Geometry check sheet. Reference: the model listing, model coordinates, mm. Face numbers are marked on the shaded views. A direction names the side the tool comes from. Give positions to 0.01 mm unless a question says otherwise; leave off trailing zeros. Order: outer loops, then holes, each group sorted by start corner. A loop starts at its lowest first (then second) coordinate and runs counter-clockwise, first axis right, second up. Notation, with made-up numbers: (-33, 67) - (-6, 67) arc R27 ccw to (-6, 98) - close; hole circle Ø5 at (-3.75, 8.5). An arc over 180 degrees is marked (long way). Put each result on its own line as item: value. Start each with the question number.
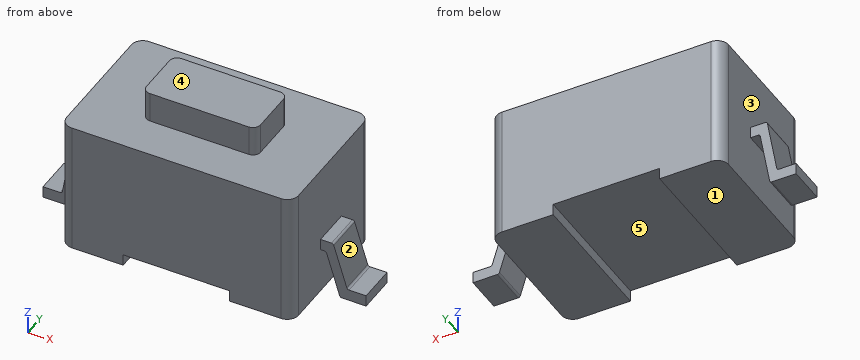
```python
from build123d import *

# Parameters (mm, degrees)
SKETCH001_W  = 6.1
SKETCH001_H  = 3.7
PAD001_DEPTH = 3.5
SKETCH002_W  = 2.8
SKETCH002_H  = 3.7
POCKET_DEPTH = 0.3
FILLET_R     = 0.3
SKETCH003_W  = 3
SKETCH003_H  = 1.5
PAD002_DEPTH = 0.8
FILLET001_R  = 0.2
PAD_DEPTH    = 0.5


with BuildPart() as obj1:
    # Sketch001 → Pad001 (new body)
    with BuildSketch(Plane.XY):
        Rectangle(SKETCH001_W, SKETCH001_H)
    extrude(amount=PAD001_DEPTH)

    # Sketch002 → Pocket (cut)
    with BuildSketch(Plane(origin=(0, 0, 0), x_dir=(1, 0, 0), z_dir=(0, 0, -1))):
        Rectangle(SKETCH002_W, SKETCH002_H)
    extrude(amount=-POCKET_DEPTH, mode=Mode.SUBTRACT)

    # Fillet
    fillet_edges = [obj1.edges().sort_by_distance(p)[0] for p in [
        (-3.05, -1.85, 1.75),
        (-3.05, 1.85, 1.75),
        (3.05, -1.85, 1.75),
        (3.05, 1.85, 1.75),
    ]]
    fillet(fillet_edges, radius=FILLET_R)

    # Sketch003 → Pad002 (new body)
    with BuildSketch(Plane.XY.offset(3.5)):
        Rectangle(SKETCH003_W, SKETCH003_H)
    extrude(amount=PAD002_DEPTH)

    # Fillet001
    fillet001_edges = [obj1.edges().sort_by_distance(p)[0] for p in [
        (1.5, -0.75, 3.9),
        (1.5, 0.75, 3.9),
        (-1.5, 0.75, 3.9),
        (-1.5, -0.75, 3.9),
    ]]
    fillet(fillet001_edges, radius=FILLET001_R)


with BuildPart() as fusion:
    # Sketch → Pad (new body, symmetric)
    with BuildSketch(Plane.XZ):
        with BuildLine():
            Line((4.25, 0), (4.25, 0.3))
            Line((4.25, 0.3), (3.8, 0.3))
            ThreePointArc((3.742663, 0.342323), (3.764367, 0.311727), (3.8, 0.3))
            Line((3.742663, 0.342323), (3.398806, 1.457677))
            ThreePointArc((3.398806, 1.457677), (3.377102, 1.488273), (3.341469, 1.5))
            Line((3.341469, 1.5), (3.05, 1.5))
            Line((3.05, 1.5), (3.05, 1.2))
            Line((3.153657, 1.2), (3.05, 1.2))
            ThreePointArc((3.210994, 1.157677), (3.18929, 1.188273), (3.153657, 1.2))
            Line((3.554852, 0.042323), (3.210994, 1.157677))
            ThreePointArc((3.554852, 0.042323), (3.576556, 0.011727), (3.612189, 0))
            Line((4.25, 0), (3.612189, 0))
        make_face()
        with BuildLine():
            Line((-3.05, 1.5), (-3.05, 1.8))
            Line((-3.434818, 1.8), (-3.05, 1.8))
            ThreePointArc((-3.434818, 1.8), (-3.473385, 1.785963), (-3.493906, 1.750419))
            Line((-3.740912, 0.349581), (-3.493906, 1.750419))
            ThreePointArc((-3.8, 0.3), (-3.761433, 0.314037), (-3.740912, 0.349581))
            Line((-4.25, 0.3), (-3.8, 0.3))
            Line((-4.25, 0), (-4.25, 0.3))
            Line((-4.25, 0), (-3.612189, 0))
            ThreePointArc((-3.612189, 0), (-3.573621, 0.014037), (-3.5531, 0.049581))
            Line((-3.5531, 0.049581), (-3.306095, 1.450419))
            ThreePointArc((-3.247006, 1.5), (-3.285573, 1.485963), (-3.306095, 1.450419))
            Line((-3.247006, 1.5), (-3.05, 1.5))
        make_face()
    extrude(amount=PAD_DEPTH, both=True)

    # Fusion: union obj1
    add(obj1.part)


solid = fusion.part
```
Item 1: Release check for a two-part mould opening along X. For the marked faces 1, 2 and 3 record: +X half, -X half, draft (parallel to the pull), parting line (faces both ways), or undercut.
Item 2: Gauge pin test, flat ends, axial feed: pin 1 Ø1.3 at (x, z) = (-3.5, 0.5) entering from +Y; pin 2 Ø0.6 at (x, z) = (-4, 0.5) entering from -Y; pin 3 Ø2 at (x, y) = (0, 0.5) entering from -Z; pin 4 Ø2 at (x, z) = (-3, 0.5) entering from -Y. Record the tip position at first contact, or that the pin passes through.
Item 3: Thickness scan on line 1 along X through (y, z) = (0.35, 0.45); line 2 along X through (y, z) = (1.05, 3.45); line 3 along Z through (x, y) = (-3, 0.4). Record the ranges inside material, lowest first.
Item 4: Cross-section at A-A (z = 3.6). Enter the section's corners in (x, y), and give its area (3 significant figures).
Item 5: Set-up check for the marked faces 4 and 5: record each of +Z, -Z, +X, -X, +Y, -Y from which the full face is reachable in a straight line by a thin tool's end or side.
Item 6: Cross-section at D-D (x = 2). Enter the section's corners in (y, z).
Item 7: Cross-section at B-B (y = -0.95). Enter the section's corners in (x, z), and give its area (3 significant figures).
Item 8: Cross-section at C-C (z = 0.5). Enter the section's corners in (x, y), and give its area (3 significant figures).
Recorded:
1. face 1: draft
1. face 2: +X half
1. face 3: undercut
2. pin 1: stops at y = 1.83
2. pin 2: stops at y = -0.5
2. pin 3: stops at z = 0.3
2. pin 4: stops at y = -1.85
3. line 1: x = -3.72 to -3.48, -3.05 to 3.05, 3.43 to 3.71
3. line 2: x = -3.05 to 3.05
3. line 3: z = 0 to 3.5
4. outline: (-1.5, -0.55) arc R0.2 ccw to (-1.3, -0.75) - (1.3, -0.75) arc R0.2 ccw to (1.5, -0.55) - (1.5, 0.55) arc R0.2 ccw to (1.3, 0.75) - (-1.3, 0.75) arc R0.2 ccw to (-1.5, 0.55) - close
4. area: 4.47 mm^2
5. face 4: +Z, +X, -X, +Y, -Y
5. face 5: -Z, +Y, -Y
6. outline: (-1.85, 0) - (1.85, 0) - (1.85, 3.5) - (-1.85, 3.5) - close
7. outline: (-3.05, 0) - (-1.4, 0) - (-1.4, 0.3) - (1.4, 0.3) - (1.4, 0) - (3.05, 0) - (3.05, 3.5) - (-3.05, 3.5) - close
7. area: 20.5 mm^2
8. outline: (-3.71, -0.5) - (-3.47, -0.5) - (-3.47, 0.5) - (-3.71, 0.5) - close; (-3.05, -1.55) arc R0.3 ccw to (-2.75, -1.85) - (2.75, -1.85) arc R0.3 ccw to (3.05, -1.55) - (3.05, 1.55) arc R0.3 ccw to (2.75, 1.85) - (-2.75, 1.85) arc R0.3 ccw to (-3.05, 1.55) - close; (3.41, -0.5) - (3.69, -0.5) - (3.69, 0.5) - (3.41, 0.5) - close
8. area: 23.0 mm^2
